from build123d import *

# Parameters (mm, degrees)
F0_W     = 21.85
F0_H     = 9.2
F1_DEPTH = 10.6
F2_W     = 0.5
F2_H     = 9.2
F3_DEPTH = 0.4


with BuildPart() as f1:
    # F0 (on Top) → F1 (new body)
    with BuildSketch(Plane.XY):
        Rectangle(F0_W, F0_H)
    extrude(amount=F1_DEPTH)

    # F2 (on face) → F3 (join)
    with BuildSketch(Plane(origin=(0, 0, 0), x_dir=(1, 0, 0), z_dir=(0, 0, -1))):
        with Locations((-10.675, 0)):
            Rectangle(F2_W, F2_H)
        with Locations((10.675, 0)):
            Rectangle(F2_W, F2_H)
    extrude(amount=F3_DEPTH)


solid = f1.part
Geometry check sheet. Reference: the model listing, model coordinates, mm. Round coordinates to 2 decimals unless told otherwise and drop trailing zeros. Order: outer loops, then holes, each group sorted by start corner. A loop starts at its lowest first (then second) coordinate and runs counter-clockwise, first axis right, second up. Notation, with made-up numbers: (74.25, 75) - (112.25, 75) arc R15 ccw to (112.25, 82) - close; hole circle Ø5 at (36.25, -21). An arc over 180 degrees is marked (long way). One line per question, with ' | ' between items. Start each with the question number.
(1) Release check for a two-part mould opening along X. For faces 1 (the flat face through (-10.925, 0, 5)), 2 (the flat face through (0, 0, 10.6)), 3 (the flat face through (0, 0, 0)), 4 (the flat face through (10.925, 0, 5)) record: released by +X, released by -X, zero draft, split by the parting line, or undercut.
(2) Sectioned sample at A-A on y = 0.75. Record the cut outline in (x, z) (3 decimals).
(3) Thickness scan on L1, parallel to Z at x = 4.75, y = 3.5. Record the ranges inside material, lowest first. Write a range as [from, to].
(4) Depth check by flat-ended pin: pin 1 Ø4.5 at (x, y) = (-1.5, 1.5) entering from -Z. Enter the tip coordinate at first touch or a pass-through.
(5) Sectioned sample at B-B on x = -0.25. Record the cut outline in (y, z).
Conclusion:
1) face 1: released by -X | face 2: zero draft | face 3: undercut | face 4: released by +X
2) outline: (-10.925, -0.4) - (-10.425, -0.4) - (-10.425, 0) - (10.425, 0) - (10.425, -0.4) - (10.925, -0.4) - (10.925, 10.6) - (-10.925, 10.6) - close
3) L1: z = [0, 10.6]
4) pin 1: stops at z = 0
5) outline: (-4.6, 0) - (4.6, 0) - (4.6, 10.6) - (-4.6, 10.6) - close
